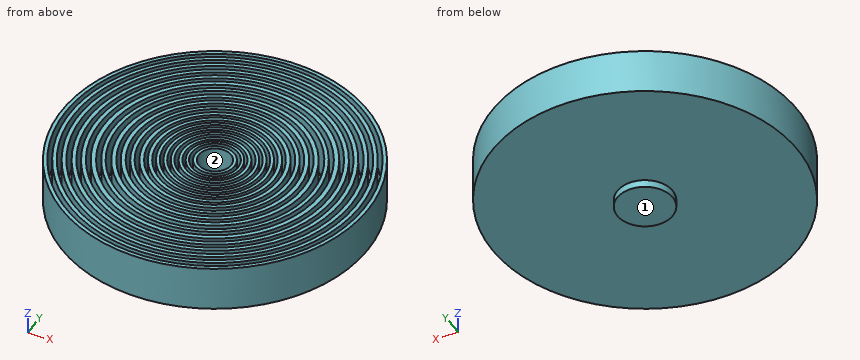
from build123d import *

# Parameters (mm, degrees)
F0_R     = 100
F1_DEPTH = 5
F2_R     = 100
F2_R_2   = 97.451659
F2_R_3   = 94.648736
F2_R_4   = 91.967315
F2_R_5   = 89.150846
F2_R_6   = 86.396715
F2_R_7   = 83.359675
F2_R_8   = 80.564885
F2_R_9   = 77.876548
F2_R_10  = 75.053444
F2_R_11  = 72.252886
F2_R_12  = 69.121186
F2_R_13  = 66.16217
F2_R_14  = 63.570133
F2_R_15  = 60.296805
F2_R_16  = 57.367289
F2_R_17  = 54.797723
F2_R_18  = 51.923775
F2_R_19  = 49.271752
F2_R_20  = 46.728635
F2_R_21  = 43.956422
F2_R_22  = 41.231373
F2_R_23  = 39.032675
F2_R_24  = 36.487368
F2_R_25  = 34.312217
F2_R_26  = 32.074481
F2_R_27  = 29.962907
F2_R_28  = 27.776258
F2_R_29  = 25.70102
F2_R_30  = 23.568539
F2_R_31  = 21.149646
F2_R_32  = 18.92981
F2_R_33  = 17.040575
F2_R_34  = 15.089483
F2_R_35  = 12.77456
F2_R_36  = 10.548498
F3_DEPTH = 25
F4_R     = 18.196703
F5_DEPTH = 5


with BuildPart() as f1:
    # F0 (on Top) → F1 (new body)
    with BuildSketch(Plane.XY):
        Circle(F0_R)
    extrude(amount=F1_DEPTH)

    # F2 (on face) → F3 (join)
    with BuildSketch(Plane.XY.offset(5)):
        Circle(F2_R)
        Circle(F2_R_2, mode=Mode.SUBTRACT)
        Circle(F2_R_3)
        Circle(F2_R_4, mode=Mode.SUBTRACT)
        Circle(F2_R_5)
        Circle(F2_R_6, mode=Mode.SUBTRACT)
        Circle(F2_R_7)
        Circle(F2_R_8, mode=Mode.SUBTRACT)
        Circle(F2_R_9)
        Circle(F2_R_10, mode=Mode.SUBTRACT)
        Circle(F2_R_11)
        Circle(F2_R_12, mode=Mode.SUBTRACT)
        Circle(F2_R_13)
        Circle(F2_R_14, mode=Mode.SUBTRACT)
        Circle(F2_R_15)
        Circle(F2_R_16, mode=Mode.SUBTRACT)
        Circle(F2_R_17)
        Circle(F2_R_18, mode=Mode.SUBTRACT)
        Circle(F2_R_19)
        Circle(F2_R_20, mode=Mode.SUBTRACT)
        Circle(F2_R_21)
        Circle(F2_R_22, mode=Mode.SUBTRACT)
        Circle(F2_R_23)
        Circle(F2_R_24, mode=Mode.SUBTRACT)
        Circle(F2_R_25)
        Circle(F2_R_26, mode=Mode.SUBTRACT)
        Circle(F2_R_27)
        Circle(F2_R_28, mode=Mode.SUBTRACT)
        Circle(F2_R_29)
        Circle(F2_R_30, mode=Mode.SUBTRACT)
        Circle(F2_R_31)
        Circle(F2_R_32, mode=Mode.SUBTRACT)
        Circle(F2_R_33)
        Circle(F2_R_34, mode=Mode.SUBTRACT)
        Circle(F2_R_35)
        Circle(F2_R_36, mode=Mode.SUBTRACT)
    extrude(amount=F3_DEPTH)

    # F4 (on face) → F5 (join)
    with BuildSketch(Plane(origin=(0, 0, 0), x_dir=(1, 0, 0), z_dir=(0, 0, -1))):
        Circle(F4_R)
    extrude(amount=F5_DEPTH)


solid = f1.part
Could you check a few things on this model? Use its own coordinates, in mm. Face numbers are marked on the shaded views. A direction names the side the tool comes from. Give positions to 0.01 mm unless a question says otherwise; leave off trailing zeros.
1. For pin 1 (4 mm diameter, centred on y = -24, z = 12.5, fed in from +X); pin 2 (6 mm diameter, centred on y = 12, z = 0, fed in from +X); pin 3 (2 mm diameter, centred on y = 58.5, z = 9, fed in from -X), each with a flat end and sliding along its axis, tell me the tip position at first contact or that it passes through.
Answers below:
pin 1: stops at x = 97.55
pin 2: stops at x = 99.59
pin 3: stops at x = -81.82
2. Suppose I cut it at A-A (z = 8). State how many separate pieces and enclosed holes the cut face has, plus the area to 3 significant figures.
Answers below:
separate pieces: 18
enclosed holes: 18
area: 15,900 mm2
3. Which directions (+Z, -Z, +X, -X, +Y, -Y) give clear straight access to the entire face, cutting with the end or side of a thin tool? Please do the marked faces 1 and 2.
Answers below:
face 1: -Z, +X, -X, +Y, -Y
face 2: +Z
4. I need wall thicknesses on L1, parallel to Z at x = -88.5, y = 3; L2, parallel to Z at x = 29.5, y = 56; L3, parallel to X at y = 57.5, z = 2.5. Which ranges of each line are inside material? Lowest first, please.
Answers below:
L1: z = 0 to 30
L2: z = 0 to 5
L3: x = -81.82 to 81.82
